Model file for the job. Use its own axes, mm. Face numbers are marked on the shaded views. A direction names the side the tool comes from. Round coordinates to 2 decimals unless told otherwise and drop trailing zeros. Order: outer loops, then holes, each group sorted by start corner. A loop starts at its lowest first (then second) coordinate and runs counter-clockwise, first axis right, second up. Notation, with made-up numbers: (-35, 45.25) - (-27, 45.25) arc R26 cw to (-27, 72.25) - close; hole circle Ø2 at (-18.75, 65). An arc over 180 degrees is marked (long way). Put each result on its own line as item: value. Start each with the question number.
Item 1: Which spindle directions (+Z, -Z, +X, -X, +Y, -Y) get a long thin tool onto all of the face, cutting with end or side? Do the marked faces 1 and 2. Say none if no direction does.
Item 2: Probe probe 1 along Z at (x, y) = (33, 19); probe 2 along Y at (x, z) = (14, 4.7); probe 3 along Y at (x, z) = (14, 1). List the from-to ranges inside material, lowest first.
Item 3: Pin check, flat tips, straight feed: pin 1 Ø8 at (x, y) = (20, 20.5) entering from +Z; pin 2 Ø1.3 at (x, z) = (18, 3.5) entering from +Y. Stop position of each tip, or through.
Item 4: Saw through at C-C on y = 3.5. List the corners of the cut face in (x, z), plus the area to 3 significant figures.
Item 5: Saw through at B-B on z = 4.75. List the corners of the cut face in (x, y).
Item 6: Saw through at D-D on x = 32.5. List the corners of the cut face in (y, z), plus the area to 3 significant figures.
Item 7: Saw through at A-A on x = 23. List the corners of the cut face in (y, z), plus the area to 3 significant figures.
```python
from build123d import *

# Parameters (mm, degrees)
F1_DEPTH = 1.55
F0_W     = 39.4
F0_H     = 1.9
F2_DEPTH = 6


with BuildPart() as f1:
    # F0 (on Top) → F1 (new body)
    with BuildSketch(Plane.XY):
        with BuildLine():
            Line((0, 17.4), (0, 1.9))
            Line((0, 1.9), (39.4, 1.9))
            Line((39.4, 1.9), (39.4, 17.4))
            ThreePointArc((39.4, 17.4), (35.240916, 27.440916), (25.2, 31.6))
            Line((25.2, 31.6), (14.2, 31.6))
            ThreePointArc((14.2, 31.6), (4.159084, 27.440916), (0, 17.4))
        make_face()
    extrude(amount=F1_DEPTH)

    # F0 (on Top) → F2 (join)
    with BuildSketch(Plane.XY):
        with Locations((19.7, 0.95)):
            Rectangle(F0_W, F0_H)
    extrude(amount=F2_DEPTH)


solid = f1.part
```
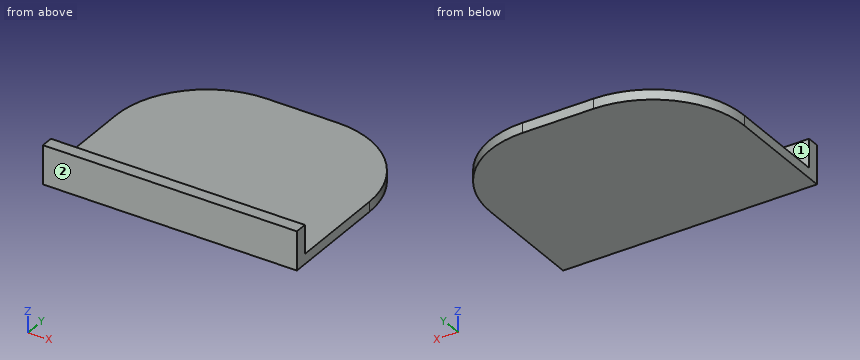
Results found:
1. face 1: +Z, +X, -X, +Y
1. face 2: +Z, -Z, +X, -X, -Y
2. probe 1: z = 0 to 1.55
2. probe 2: y = 0 to 1.9
2. probe 3: y = 0 to 31.6
3. pin 1: stops at z = 1.55
3. pin 2: stops at y = 1.9
4. outline: (0, 0) - (39.4, 0) - (39.4, 1.55) - (0, 1.55) - close
4. area: 61.1 mm²
5. outline: (0, 0) - (39.4, 0) - (39.4, 1.9) - (0, 1.9) - close
6. outline: (0, 0) - (29.58, 0) - (29.58, 1.55) - (1.9, 1.55) - (1.9, 6) - (0, 6) - close
6. area: 54.3 mm²
7. outline: (0, 0) - (31.6, 0) - (31.6, 1.55) - (1.9, 1.55) - (1.9, 6) - (0, 6) - close
7. area: 57.4 mm²
